```python
from build123d import *

# Parameters (mm, degrees)
F0_W     = 404
F0_H     = 145
F2_DEPTH = 3
F1_R     = 2.5
F1_R_2   = 11
F1_R_3   = 1.8
F1_R_4   = 1.75
F1_W     = 53.3
F1_H     = 13
F1_W_2   = 7
F1_H_2   = 14.5
F1_R_5   = 1.5
F3_DEPTH = 25


with BuildPart() as f2:
    # F0 (on Top) → F2 (new body)
    with BuildSketch(Plane.XY):
        with Locations((-14.1859020234, -7.6260944492)):
            Rectangle(F0_W, F0_H)
    extrude(amount=-F2_DEPTH)

    # F1 (on Top) → F3 (cut)
    with BuildSketch(Plane.XY):
        with Locations((-210.1859020234, -68.1260944492)):
            Circle(F1_R)
        with BuildLine():
            Line((-135.1859020234, 49.1823275357), (-135.1859020234, 40.5654835659))
            ThreePointArc((-135.1859020234, 40.5654835659), (-128.3859020234, 36.8239055508), (-121.5859020234, 40.5654835659))
            Line((-121.5859020234, 40.5654835659), (-121.5859020234, 49.1823275357))
            ThreePointArc((-121.5859020234, 49.1823275357), (-128.3859020234, 52.9239055508), (-135.1859020234, 49.1823275357))
        make_face()
        with BuildLine():
            ThreePointArc((-22.25, -52.9147846764), (-11.3343496313, -46.8414689631), (-7, -35.1260944492))
            ThreePointArc((-7, -35.1260944492), (-36.7153745139, -21.4604440805), (-27.75, -52.9147846764))
            Line((-27.75, -52.9147846764), (-27.75, -31.4030106551))
            Line((-27.75, -31.4030106551), (-22.25, -31.4030106551))
            Line((-22.25, -31.4030106551), (-22.25, -52.9147846764))
        make_face()
        with BuildLine():
            Line((-27.75, -31.4030106551), (-27.75, -52.9147846764))
            ThreePointArc((-27.75, -52.9147846764), (-25, -53.1260944492), (-22.25, -52.9147846764))
            Line((-22.25, -52.9147846764), (-22.25, -31.4030106551))
            Line((-22.25, -31.4030106551), (-27.75, -31.4030106551))
        make_face()
        with BuildLine():
            ThreePointArc((-22.25, -52.9147846764), (-25, -53.1260944492), (-27.75, -52.9147846764))
            Line((-27.75, -52.9147846764), (-27.75, -56.6260944492))
            Line((-27.75, -56.6260944492), (-22.25, -56.6260944492))
            Line((-22.25, -56.6260944492), (-22.25, -52.9147846764))
        make_face()
        with Locations((-25, 44.8739055508)):
            Circle(F1_R_2)
        with Locations((-40.5, 44.8739055508)):
            Circle(F1_R_3)
        with Locations((-9.5, 44.8739055508)):
            Circle(F1_R_3)
        with Locations((-210.1859020234, -48.1260944492)):
            Circle(F1_R)
        with BuildLine():
            Line((152.8140979766, 39.8739055508), (172.8140979766, 39.8739055508))
            ThreePointArc((172.8140979766, 39.8739055508), (175.6425251014, 41.045478426), (176.8140979766, 43.8739055508))
            Line((176.8140979766, 43.8739055508), (176.8140979766, 55.8739055508))
            ThreePointArc((176.8140979766, 55.8739055508), (175.6425251014, 58.7023326755), (172.8140979766, 59.8739055508))
            Line((172.8140979766, 59.8739055508), (152.8140979766, 59.8739055508))
            ThreePointArc((152.8140979766, 59.8739055508), (149.9856708519, 58.7023326755), (148.8140979766, 55.8739055508))
            Line((148.8140979766, 55.8739055508), (148.8140979766, 43.8739055508))
            ThreePointArc((148.8140979766, 43.8739055508), (149.9856708519, 41.045478426), (152.8140979766, 39.8739055508))
        make_face()
        with Locations((142.8140979766, 49.8739055508)):
            Circle(F1_R_4)
        with Locations((182.8140979766, 49.8739055508)):
            Circle(F1_R_4)
        with Locations((-174.0359020234, -51.6260944492)):
            Rectangle(F1_W, F1_H)
        with Locations((-114.3359020234, -51.6260944492)):
            Rectangle(F1_W, F1_H)
        with Locations((-200.6859020234, 44.8239055508)):
            Rectangle(F1_W_2, F1_H_2)
        with Locations((-200.6859020234, 59.8739055508)):
            Circle(F1_R_5)
        with Locations((-200.6859020234, 29.7739055508)):
            Circle(F1_R_5)
        with Locations((-173.6859020234, 44.8239055508)):
            Rectangle(F1_W_2, F1_H_2)
        with Locations((-173.6859020234, 59.8739055508)):
            Circle(F1_R_5)
        with Locations((-173.6859020234, 29.7739055508)):
            Circle(F1_R_5)
        with BuildLine():
            Line((-91.5859020234, 49.1823275357), (-91.5859020234, 40.5654835659))
            ThreePointArc((-91.5859020234, 40.5654835659), (-84.7859020234, 36.8239055508), (-77.9859020234, 40.5654835659))
            Line((-77.9859020234, 40.5654835659), (-77.9859020234, 49.1823275357))
            ThreePointArc((-77.9859020234, 49.1823275357), (-84.7859020234, 52.9239055508), (-91.5859020234, 49.1823275357))
        make_face()
        with Locations((-201.1859020234, -65.1260944492)):
            Circle(F1_R_5)
        with Locations((-87.1859020234, -65.1260944492)):
            Circle(F1_R_5)
    extrude(amount=-F3_DEPTH, mode=Mode.SUBTRACT)


solid = f2.part
```
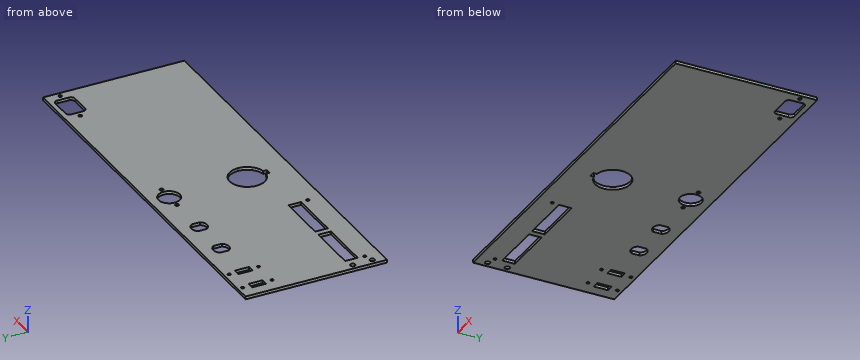
Work out the finished part from the listing and answer in its coordinate system (mm). Round coordinates to 2 decimals unless told otherwise and drop trailing zeros. Loops run counter-clockwise (first coordinate to the right, second up) from the corner with the lowest first, then second, coordinate; pieces in that order, holes last.
(1) This flat-tipped pin is pushed along its axis until it touches: P1, Ø3, axis at x = 182.81, y = 49.87, coming from the +Z side. Where does it stop, or does it pass through?
Computed values:
P1: passes through
(2) The part is cut by section A-A, the plane y = -25. Give the vertices of the cut face in (x, z), and give its area (3 significant figures).
Computed values:
outline: (-216.19, -3) - (-39.88, -3) - (-39.88, 0) - (-216.19, 0) - close; (-10.12, -3) - (187.81, -3) - (187.81, 0) - (-10.12, 0) - close
area: 1,120 mm2
(3) The part is cut by section B-B, the plane z = -1.25. Give the number of separate pieces and of enclosed holes in the cut face, and give its area (3 significant figures).
Computed values:
separate pieces: 1
enclosed holes: 21
area: 54,500 mm2
(4) Find the intervals of material crossed by L1, parallel to X at y = -54, z = -1.6; L2, parallel to Y at x = -25, z = -1.65; L3, parallel to Y at x = -174, z = -1.95, in increasing order.
Computed values:
L1: x = -216.19 to -200.69, -147.39 to -140.99, -87.69 to -27.75, -22.25 to 187.81
L2: y = -80.13 to -56.63, -17.13 to 33.87, 55.87 to 64.87
L3: y = -80.13 to -58.13, -45.13 to 28.31, 31.24 to 37.57, 52.07 to 58.41, 61.34 to 64.87
